```python
from build123d import *

# Parameters (mm, degrees)
SKETCH1_R           = 12.2
SKETCH1_R_2         = 1.5
BOSS_EXTRUDE1_DEPTH = 7
SKETCH2_R           = 12.2
SKETCH2_R_2         = 10
BOSS_EXTRUDE2_DEPTH = 2
SKETCH3_R           = 3
CUT_EXTRUDE1_DEPTH  = 2
SKETCH4_R           = 3
CUT_EXTRUDE2_DEPTH  = 2


with BuildPart() as part:
    # Sketch1 → Boss-Extrude1 (new body)
    with BuildSketch(Plane(origin=(0, 0, 0), x_dir=(1, 0, 0), z_dir=(0, 1, 0))):
        Polygon((-12, 22), (-12, 13), (12, 13), (12, 22), (35, 22), (35, -22), (-35, -22), (-35, 22), align=None)
        with Locations(Location((0, 0, 0), (0, 0, 270))):
            Circle(SKETCH1_R, mode=Mode.SUBTRACT)
        with Locations(Location((27.5, -15, 0), (0, 0, 270))):
            Circle(SKETCH1_R_2, mode=Mode.SUBTRACT)
        with Locations(Location((27.5, 15, 0), (0, 0, 270))):
            Circle(SKETCH1_R_2, mode=Mode.SUBTRACT)
        with Locations(Location((-27.5, -15, 0), (0, 0, 270))):
            Circle(SKETCH1_R_2, mode=Mode.SUBTRACT)
        with Locations(Location((-27.5, 15, 0), (0, 0, 270))):
            Circle(SKETCH1_R_2, mode=Mode.SUBTRACT)
        with Locations(Location((15.5, -15.5, 0), (0, 0, 270))):
            Circle(SKETCH1_R_2, mode=Mode.SUBTRACT)
        with Locations(Location((-15.5, -15.5, 0), (0, 0, 270))):
            Circle(SKETCH1_R_2, mode=Mode.SUBTRACT)
        with Locations(Location((15.5, 15.5, 0), (0, 0, 270))):
            Circle(SKETCH1_R_2, mode=Mode.SUBTRACT)
        with Locations(Location((-15.5, 15.5, 0), (0, 0, 270))):
            Circle(SKETCH1_R_2, mode=Mode.SUBTRACT)
    extrude(amount=BOSS_EXTRUDE1_DEPTH)

    # Sketch2 → Boss-Extrude2 (add)
    with BuildSketch(Plane.XZ):
        with Locations(Location((0, 0, 0), (0, 0, 270))):
            Circle(SKETCH2_R)
        with Locations(Location((0, 0, 0), (0, 0, 270))):
            Circle(SKETCH2_R_2, mode=Mode.SUBTRACT)
    extrude(amount=-BOSS_EXTRUDE2_DEPTH)

    # Sketch3 → Cut-Extrude1 (cut)
    with BuildSketch(Plane.XZ):
        with Locations(Location((-27.5, 15, 0), (0, 0, 270))):
            Circle(SKETCH3_R)
        with Locations(Location((-27.5, -15, 0), (0, 0, 270))):
            Circle(SKETCH3_R)
        with Locations(Location((27.5, 15, 0), (0, 0, 270))):
            Circle(SKETCH3_R)
        with Locations(Location((27.5, -15, 0), (0, 0, 270))):
            Circle(SKETCH3_R)
    extrude(amount=-CUT_EXTRUDE1_DEPTH, mode=Mode.SUBTRACT)

    # Sketch4 → Cut-Extrude2 (cut)
    with BuildSketch(Plane(origin=(0, 7, 0), x_dir=(1, 0, 0), z_dir=(0, 1, 0))):
        with Locations(Location((15.5, -15.5, 0), (0, 0, 270))):
            Circle(SKETCH4_R)
        with Locations(Location((-15.5, -15.5, 0), (0, 0, 270))):
            Circle(SKETCH4_R)
        with Locations(Location((15.5, 15.5, 0), (0, 0, 270))):
            Circle(SKETCH4_R)
        with Locations(Location((-15.5, 15.5, 0), (0, 0, 270))):
            Circle(SKETCH4_R)
    extrude(amount=-CUT_EXTRUDE2_DEPTH, mode=Mode.SUBTRACT)


solid = part.part
```
Design review of the part built by this model. Coordinates are the model's own, in mm. A direction names the side the tool comes from. Give positions to 0.01 mm unless a question says otherwise; leave off trailing zeros. Write each loop counter-clockwise with the first axis right and the second up, starting at its lowest first coordinate (ties: lowest second). Pieces come first, ordered by that corner, then holes. Notation, with made-up numbers: (75, 6.5) -> (95, 6.5) arc R17 cw to (95, 37.5) -> close; hole circle Ø8 at (-2, 19). An arc over 180 degrees is marked (long way). Answer in a Markdown table with one row per item.
(1) Consider section D-D (z = -8.5). State the section outline as (x, y) points.
Results:
| item | result |
|---|---|
| outline | (-35, 0) -> (-5.27, 0) -> (-5.27, 2) -> (-8.75, 2) -> (-8.75, 7) -> (-35, 7) -> close; (5.27, 0) -> (35, 0) -> (35, 7) -> (8.75, 7) -> (8.75, 2) -> (5.27, 2) -> close |
(2) Mouldability with a two-part tool opening along X and no side actions: class faces 1 (the flat face through (8.3, 7, 9.5)), 2 (the flat face through (-17, 5, 17)) as +X half, -X half, draft (parallel to the pull), parting line (faces both ways), or undercut.
Results:
| item | result |
|---|---|
| face 1 | draft |
| face 2 | undercut |
(3) For faces 3 (the flat face through (-26, 2, -16)), 4 (the flat face through (12, 3, -17)), 5 (the cylindrical face through (-26.49, 4.46, -16.11)), 6 (the cylindrical face through (-7.4, 4.5, -9.7)), list the 3-axis set-ups (+Z, -Z, +X, -X, +Y, -Y) from which the entire face can be reached by the end or side of a thin tool; tool diameter is ignored.
Results:
| item | result |
|---|---|
| face 3 | -Y |
| face 4 | -Z, +Y, -Y |
| face 5 | +Y, -Y |
| face 6 | +Y |
(4) To check wall thickness, follow probe 1 along Z at (x, y) = (-27.5, 3.9); probe 2 along X at (y, z) = (5, -19.5); probe 3 along Z at (x, y) = (-18, 5.75). State the ranges of each line that lie inside material, in increasing order.
Results:
| item | result |
|---|---|
| probe 1 | -22 to -16.5, -13.5 to 13.5, 16.5 to 22 |
| probe 2 | -35 to -12, 12 to 35 |
| probe 3 | -22 to -17.16, -13.84 to 13.84, 17.16 to 22 |
(5) Consider section C-C (x = 0). State the section outline as (y, z) points.
Results:
| item | result |
|---|---|
| outline | (0, -13) -> (7, -13) -> (7, -12.2) -> (2, -12.2) -> (2, -10) -> (0, -10) -> close; (0, 10) -> (2, 10) -> (2, 12.2) -> (7, 12.2) -> (7, 22) -> (0, 22) -> close |
(6) Consider section B-B (y = 6). Count the separate pieces of the cut face and the enclosed holes in it, then the cut area to 3 significant figures.
Results:
| item | result |
|---|---|
| separate pieces | 1 |
| enclosed holes | 9 |
| area | 2,260 mm2 |
(7) Clearance check with flat-ended pins moving along their axes: pin 1 (1.8 mm diameter, centred on x = -17, z = 16, fed in from +Y); pin 2 (2.5 mm diameter, centred on x = -27.5, z = -15, fed in from -Y); pin 3 (2 mm diameter, centred on x = 9, y = 1, fed in from -Z); pin 4 (1 mm diameter, centred on x = -10, z = 3, fed in from +Y). State where each tip first meets the part, or that it passes through.
Results:
| item | result |
|---|---|
| pin 1 | y = 5 |
| pin 2 | through |
| pin 3 | z = -13 |
| pin 4 | y = 2 |
(8) Consider section A-A (x = -27.5). State the section outline as (y, z) points, then the cut area to 3 significant figures.
Results:
| item | result |
|---|---|
| outline | (0, -22) -> (7, -22) -> (7, -16.5) -> (2, -16.5) -> (2, -18) -> (0, -18) -> close; (0, -12) -> (2, -12) -> (2, -13.5) -> (7, -13.5) -> (7, 13.5) -> (2, 13.5) -> (2, 12) -> (0, 12) -> close; (0, 18) -> (2, 18) -> (2, 16.5) -> (7, 16.5) -> (7, 22) -> (0, 22) -> close |
| area | 254 mm2 |
